The model under review builds one solid part; all positions refer to its coordinate system, in mm. Give positions to 0.01 mm unless a question says otherwise; leave off trailing zeros. Loops run counter-clockwise (first coordinate to the right, second up) from the corner with the lowest first, then second, coordinate; pieces in that order, holes last. Notation, with made-up numbers: (-24, 28.25) - (-9, 28.25) arc R18 cw to (-9, 48.25) - close; hole circle Ø9 at (42.5, -35). An arc over 180 degrees is marked (long way). Answer as a JSON object with one key per item and string values.
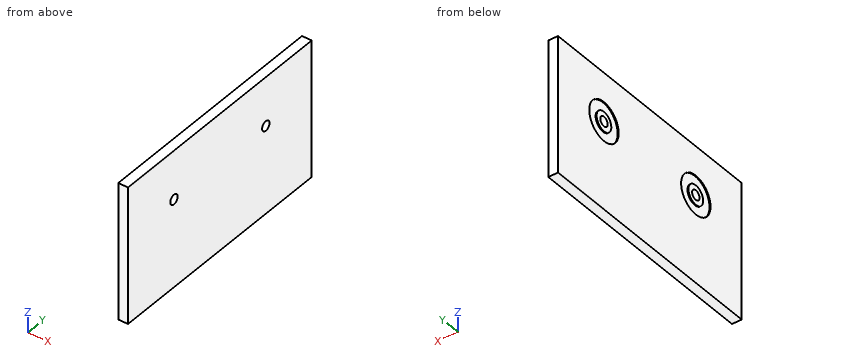
Solid Edge part; units mm, degrees
sketch "Sketch1" plane through (0, 0, 0) normal (1, 0, 0) x (0, 1, 0)
  line L0 (-80.5059, -20.8442) -> (169.4941, -20.8442)
  line L1 (169.4941, -20.8442) -> (169.4941, 119.1558)
  line L2 (169.4941, 119.1558) -> (-80.5059, 119.1558)
  line L3 (-80.5059, 119.1558) -> (-80.5059, -20.8442)
  dimension "D1" = 80.5059
  dimension "D2" = 80.5059
extrude "Protrusion1" add sketch "Sketch1" against normal blind 10
sketch "Sketch2" plane through (-10, 44.4941, 29.1558) normal (-1, 0, 0) x (0, -1, 0)
  circle A0 centre (-62.5, 40) radius 10
  circle A1 centre (62.5, 40) radius 20
  circle A2 centre (62.5, 40) radius 10
  circle A3 centre (-62.5, 40) radius 20
  dimension "D1" = 62.5
extrude "Cutout1" cut sketch "Sketch2" against normal blind 1
sketch "Sketch3" plane through (0, 44.4941, 29.1558) normal (1, 0, 0) x (0, 1, 0)
  circle A0 centre (62.5, 40) radius 5
  circle A1 centre (-62.5, 40) radius 5
extrude "Cutout2" cut sketch "Sketch3" against normal through all
Q1. To check wall thickness, follow probe 1 along Z at (x, y) = (-1.25, -14.5); probe 2 along X at (y, z) = (-6, 64.5). State the ranges of each line that lie inside material, in increasing order. Write a range as [from, to].
Results:
{"probe 1": "z = [-20.84, 65.59], [72.72, 119.16]", "probe 2": "x = [-9, 0]"}
Q2. Consider section A-A, the plane y = 124. State the section outline as (x, z) points, plus the area to 3 significant figures.
Results:
{"outline": "(-10, -20.84) - (0, -20.84) - (0, 119.16) - (-10, 119.16) - (-10, 79.68) - (-9, 79.68) - (-9, 58.63) - (-10, 58.63) - close", "area": "1,380 mm^2"}
Q3. Consider section B-B, the plane y = -25.5. State the section outline as (x, z) points.
Results:
{"outline": "(-10, -20.84) - (0, -20.84) - (0, 119.16) - (-10, 119.16) - (-10, 87.7) - (-9, 87.7) - (-9, 75.78) - (-10, 75.78) - (-10, 62.53) - (-9, 62.53) - (-9, 50.61) - (-10, 50.61) - close"}
